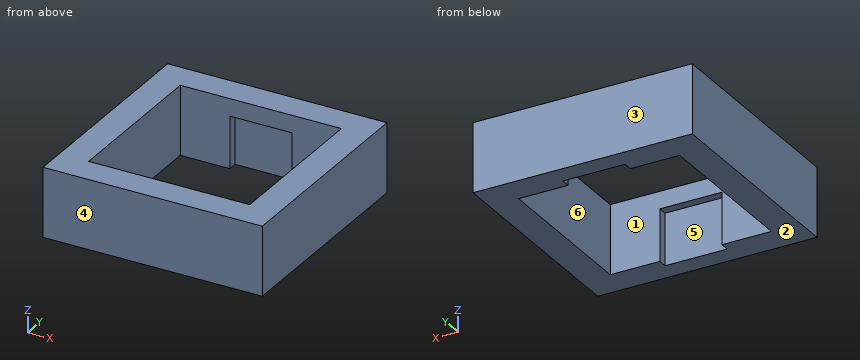
```python
from build123d import *

# Parameters (mm, degrees)
SKETCH1_W           = 19.05
SKETCH1_H           = 19.05
SKETCH1_W_2         = 14
SKETCH1_H_2         = 14
BOSS_EXTRUDE1_DEPTH = 6
CUT_EXTRUDE1_START  = -0.8
SKETCH2_W           = 5.4
SKETCH2_H           = 4.5
CUT_EXTRUDE1_DEPTH  = 15.6


with BuildPart() as part:
    # Sketch1 → Boss-Extrude1 (new body)
    with BuildSketch(Plane.XY):
        Rectangle(SKETCH1_W, SKETCH1_H)
        Rectangle(SKETCH1_W_2, SKETCH1_H_2, mode=Mode.SUBTRACT)
    extrude(amount=BOSS_EXTRUDE1_DEPTH)

    # Sketch2 → Cut-Extrude1 (cut)
    with BuildSketch(Plane.XZ.offset(-7).offset(CUT_EXTRUDE1_START)):
        with Locations((0, 2.25)):
            Rectangle(SKETCH2_W, SKETCH2_H)
    extrude(amount=CUT_EXTRUDE1_DEPTH, mode=Mode.SUBTRACT)


solid = part.part
```
Verification items for the finished model (mm, model axes). Face numbers are marked on the shaded views. A direction names the side the tool comes from. Coordinates: 2 decimals unless noted, no trailing zeros. Order: outer loops, then holes, each group sorted by start corner. A loop starts at its lowest first (then second) coordinate and runs counter-clockwise, first axis right, second up. Notation, with made-up numbers: (39.5, -27.75) -> (64.5, -27.75) arc R25 cw to (64.5, 1.25) -> close; hole circle Ø4 at (-10, -25). An arc over 180 degrees is marked (long way). Answer as CSV lines item,"result". Start each with the question number.
1) Cross-section at A-A, the plane x = -6.75. Record the boundary of the cut face in (y, z) (3 decimals).
2) Release check for a two-part mould opening along Y. For the marked faces 1, 2 and 3 record: released by +Y, released by -Y, zero draft, split by the parting line, or undercut.
3) Material ranges on L1, parallel to Y at x = 2.25, z = 0.6 (3 decimals); L2, parallel to X at y = 2.75, z = 5.55 (3 decimals); L3, parallel to X at y = -7.5, z = 0.9 (3 decimals), recorded low to high. Write a range as [from, to].
4) Set-up check for the marked faces 4, 5 and 6: record each of +Z, -Z, +X, -X, +Y, -Y from which the full face is reachable in a straight line by a thin tool's end or side.
5) Cross-section at D-D, the plane x = -0.25. Record the boundary of the cut face in (y, z) (3 decimals).
6) Cross-section at C-C, the plane z = 2.05. Record the boundary of the cut face in (x, y) (3 decimals), then the cut area to 3 significant figures.
Conclusion:
1,outline,"(-9.525, 0) -> (-7, 0) -> (-7, 6) -> (-9.525, 6) -> close; (7, 0) -> (9.525, 0) -> (9.525, 6) -> (7, 6) -> close"
2,face 1,"undercut"
2,face 2,"zero draft"
2,face 3,"released by +Y"
3,L1,"y = [-9.525, -7.8], [7.8, 9.525]"
3,L2,"x = [-9.525, -7], [7, 9.525]"
3,L3,"x = [-9.525, -2.7], [2.7, 9.525]"
4,face 4,"+Z, -Z, +X, -X, -Y"
4,face 5,"-Z"
4,face 6,"+Z, -Z"
5,outline,"(-9.525, 0) -> (-7.8, 0) -> (-7.8, 4.5) -> (-7, 4.5) -> (-7, 6) -> (-9.525, 6) -> close; (7, 4.5) -> (7.8, 4.5) -> (7.8, 0) -> (9.525, 0) -> (9.525, 6) -> (7, 6) -> close"
6,outline,"(-9.525, -9.525) -> (9.525, -9.525) -> (9.525, 9.525) -> (-9.525, 9.525) -> close; hole (-7, -7) -> (-2.7, -7) -> (-2.7, -7.8) -> (2.7, -7.8) -> (2.7, -7) -> (7, -7) -> (7, 7) -> (2.7, 7) -> (2.7, 7.8) -> (-2.7, 7.8) -> (-2.7, 7) -> (-7, 7) -> close"
6,area,"158 mm²"
